Autodesk Inventor part; units mm, degrees
ref_plane "YZ Plane" through (0, 0, 0) normal (1, 0, 0) x (0, 1, 0)
ref_plane "XZ Plane" through (0, 0, 0) normal (0, 1, 0) x (-1, 0, 0)
ref_plane "XY Plane" through (0, 0, 0) normal (0, 0, 1) x (1, 0, 0)
sketch "Эскиз1" plane through (0, 0, 0) normal (0, 0, 1) x (1, 0, 0)
  line L0 (-5, -7.5) -> (5, -7.5)
  line L1 (5, -7.5) -> (5, 7.5)
  line L2 (5, 7.5) -> (-5, 7.5)
  line L3 (-5, 7.5) -> (-5, -7.5)
  line L4 (-5, -7.5) -> (5, 7.5) construction
  line L5 (5, -7.5) -> (-5, 7.5) construction
  point P0 (0, 0)
  dimension "d0" = 10
  dimension "d1" = 15
extrude "Выдавливание1" add sketch "Эскиз1" along normal mid plane 240
sketch "Эскиз3" plane through (-5, 7.5, 120) normal (0, 1, 0) x (1, 0, 0)
  line L0 (10, 0) -> (22.4133, 11.0717) construction
  line L1 (10, 240) -> (10, 0)
  line L2 (18.7544, 123.2595) -> (14.9087, 136.6513) construction
  line L3 (14.9087, 136.6513) -> (10, 148.7613) construction
  line L4 (12.2217, 156.9873) -> (15.1095, 158.4366) construction
  line L5 (10, 158.6272) -> (12.2217, 156.9873) construction
  spline S0 degree 4 poles (10, 120.3104) (10.6885, 120.4) (14.5524, 120.9622) (18.7544, 123.2595) (14.9087, 136.6513) (10, 148.7613) knots 7.806725 7.806725 7.806725 7.806725 7.806725 8 8.816044 8.816044 8.816044 8.816044 8.816044
  line L6 (16.1722, 104.0435) -> (12.6846, 108.5719) construction
  line L7 (12.6846, 108.5719) -> (10, 112.3423) construction
  line L8 (14.5524, 120.9622) -> (18.7544, 123.2595) construction
  line L9 (10.6885, 120.4) -> (14.5524, 120.9622) construction
  line L10 (10, 120.3104) -> (10.6885, 120.4) construction
  line L11 (19.5701, 51.9157) -> (11.8452, 59.5335) construction
  line L12 (11.8452, 59.5335) -> (10, 61.4441) construction
  line L13 (12.6625, 64.9164) -> (17.1948, 66.8214) construction
  line L14 (10, 64.7616) -> (12.6625, 64.9164) construction
  spline S1 degree 4 poles (10, 0) (22.4133, 11.0717) (20.5125, 21.2759) (14.9788, 29.1456) (10, 34.6409) knots 1 1 1 1 1 1.479533 1.479533 1.479533 1.479533 1.479533
  spline S2 degree 4 poles (10, 42.4578) (17.8063, 40.9171) (31.518, 38.9171) (19.5701, 51.9157) (11.8452, 59.5335) (10, 61.4441) knots 2.157548 2.157548 2.157548 2.157548 2.157548 3 3.460409 3.460409 3.460409 3.460409 3.460409
  line L15 (22.4133, 11.0717) -> (20.5125, 21.2759) construction
  line L16 (20.5125, 21.2759) -> (14.9788, 29.1456) construction
  line L17 (14.9788, 29.1456) -> (10, 34.6409) construction
  line L18 (31.518, 38.9171) -> (19.5701, 51.9157) construction
  line L19 (17.8063, 40.9171) -> (31.518, 38.9171) construction
  line L20 (10, 42.4578) -> (17.8063, 40.9171) construction
  spline S3 degree 4 poles (10, 64.7616) (12.6625, 64.9164) (17.1948, 66.8214) (12.7242, 81.5872) (10.4023, 92.5211) (10, 95.1158) knots 4.079114 4.079114 4.079114 4.079114 4.079114 5 5.351232 5.351232 5.351232 5.351232 5.351232
  spline S4 degree 4 poles (10, 102.7457) (10.3255, 103.6616) (12.3365, 106.1869) (16.1722, 104.0435) (12.6846, 108.5719) (10, 112.3423) knots 5.710697 5.710697 5.710697 5.710697 5.710697 6 6.927418 6.927418 6.927418 6.927418 6.927418
  line L21 (17.1948, 66.8214) -> (12.7242, 81.5872) construction
  line L22 (12.7242, 81.5872) -> (10.4023, 92.5211) construction
  line L23 (10.4023, 92.5211) -> (10, 95.1158) construction
  line L24 (12.3365, 106.1869) -> (16.1722, 104.0435) construction
  line L25 (10.3255, 103.6616) -> (12.3365, 106.1869) construction
  line L26 (10, 102.7457) -> (10.3255, 103.6616) construction
  spline S5 degree 4 poles (10, 158.6272) (12.2217, 156.9873) (15.1095, 158.4366) (12.3637, 173.2023) (10.5216, 183.4118) (10, 187.241) knots 10.452108 10.452108 10.452108 10.452108 10.452108 11 11.609642 11.609642 11.609642 11.609642 11.609642
  line L27 (15.1095, 158.4366) -> (12.3637, 173.2023) construction
  line L28 (12.3637, 173.2023) -> (10.5216, 183.4118) construction
  line L29 (10.5216, 183.4118) -> (10, 187.241) construction
  line L30 (10.7467, 195.0702) -> (13.4688, 194.3249) construction
  line L31 (10, 193.6844) -> (10.7467, 195.0702) construction
  spline S6 degree 4 poles (10, 193.6844) (10.7467, 195.0702) (13.4688, 194.3249) (15.4545, 200.7955) (11.7294, 208.8265) (10, 212.1471) knots 12.053463 12.053463 12.053463 12.053463 12.053463 13 13.695165 13.695165 13.695165 13.695165 13.695165
  spline S7 degree 4 poles (10, 227.67) (10.6941, 228.2247) (12.3194, 229.5337) (13.2597, 230.885) (11.5359, 232.7441) (10, 233.9261) knots 14.764065 14.764065 14.764065 14.764065 14.764065 15 15.335911 15.335911 15.335911 15.335911 15.335911
  line L32 (13.4688, 194.3249) -> (15.4545, 200.7955) construction
  line L33 (15.4545, 200.7955) -> (11.7294, 208.8265) construction
  line L34 (11.7294, 208.8265) -> (10, 212.1471) construction
  line L35 (10.6941, 228.2247) -> (12.3194, 229.5337) construction
  line L36 (10, 227.67) -> (10.6941, 228.2247) construction
  line L37 (12.3194, 229.5337) -> (13.2597, 230.885) construction
  line L38 (13.2597, 230.885) -> (11.5359, 232.7441) construction
  line L39 (11.5359, 232.7441) -> (10, 233.9261) construction
  point P0 (5, 120)
extrude "Выдавливание3" add sketch "Эскиз3" against normal blind 15
sketch "Эскиз4" plane through (-5, 7.5, -120) normal (0, 1, 0) x (1, 0, 0)
  line L0 (0, -240) -> (0, -120) construction
  line L1 (0, 0) -> (0, -240) construction
  circle A0 centre (5, -120) radius 2
  dimension "d15" = 4
extrude "Выдавливание4" cut sketch "Эскиз4" against normal blind 15
properties part number "Nozzle"
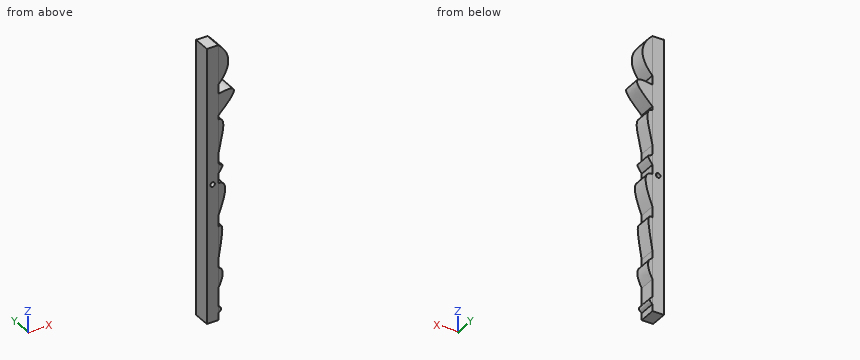
Input: part model. Units: mm. Frame: model coordinates. Coordinates: 2 decimals unless noted, no trailing zeros. Loops run counter-clockwise (first coordinate to the right, second up) from the corner with the lowest first, then second, coordinate; pieces in that order, holes last. Notation, with made-up numbers: (9.25, 88) - (52.25, 88) arc R20 cw to (52.25, 123) - close; hole circle Ø6 at (33, 43). An arc over 180 degrees is marked (long way). Answer in a Markdown table with one row per item. Add a question column.
Item 1: Section query B-B on z = -105. Return the cut outline in (x, y), then the cut area to 3 significant figures.
Item 2: Section query A-A on x = 0. Return the cut outline in (y, z).
Item 3: Line query: line 1 along X through (y, z) = (2.25, 0); line 2 along Z through (x, y) = (0, 2.75); line 3 along X through (y, z) = (4, -100.5). Output: solid intervals per line, ascending. Write a range as [from, to].
Item 4: Contact query for flat-ended pins moving along their axis: P1, Ø5, axis at y = -2, z = -34, coming from the +X side; P2, Ø6.5, axis at y = -2, z = -116, coming from the +X side; P3, Ø9, axis at y = 0, z = 3, coming from the +X side. Output: stop coordinate, or through.
Recorded:
| question | item | result |
|---|---|---|
| 1 | outline | (-5, -7.5) - (5, -7.5) - (5, 7.5) - (-5, 7.5) - close |
| 1 | area | 150 mm^2 |
| 2 | outline | (-7.5, -120) - (7.5, -120) - (7.5, -2) - (-7.5, -2) - close; (-7.5, 2) - (7.5, 2) - (7.5, 120) - (-7.5, 120) - close |
| 3 | line 1 | [-5, -2], [2, 5] |
| 3 | line 2 | [-120, -2], [2, 120] |
| 3 | line 3 | [-5, 5] |
| 4 | P1 | x = 5 |
| 4 | P2 | x = 6.35 |
| 4 | P3 | x = 8.82 |
